Input: part model. Units: mm. Frame: model coordinates. A direction names the side the tool comes from. Round coordinates to 2 decimals unless told otherwise and drop trailing zeros. Order: outer loops, then holes, each group sorted by start corner. A loop starts at its lowest first (then second) coordinate and runs counter-clockwise, first axis right, second up.
Item 1: Reachability of faces 4 (the flat face through (0, 2.75, 3)), 5 (the flat face through (41.675, 4.435, 2.958)) from +Z, -Z, +X, -X, +Y, -Y: full face, straight path, thin tool, end or side. Return the list, or none.
Item 2: Mould query, pull axis X, two halves, no side actions, for faces 1 (the flat face through (0, -2.75, 3)), 2 (the flat face through (22, 1, 6)), 3 (the flat face through (41.438, -4.565, 2.958)). Classes: released by +X, released by -X, zero draft, split by the parting line, or undercut.
Item 3: Cut plane B-B on z = 2.8. Output: boundary loops of the cut face in (x, y), then the cut area to 3 significant figures.
Item 4: First-contact query: pin 1 (1 mm diameter, centred on x = 19, z = 4, fed in from +Y); pin 2 (3 mm diameter, centred on x = 26.5, z = 1.5, fed in from -Y); pin 3 (1.8 mm diameter, centred on x = -0.5, z = 2.5, fed in from -Y); pin 4 (1.5 mm diameter, centred on x = 5.5, y = -3.5, fed in from +Z). Flat tips, straight axial feed; report the tip coordinate or a pass-through.
Item 5: Cut plane A-A on x = 0. Output: boundary loops of the cut face in (y, z).
Item 6: Line query: L1, parallel to X at y = -2.5, z = 3.25; L2, parallel to X at y = -2.25, z = 3.8; L3, parallel to Y at x = 30, z = 1.2. Output: solid intervals per line, ascending.
Item 7: Cut plane C-C on y = -2. Output: boundary loops of the cut face in (x, z), then the cut area to 3 significant figures.
Item 8: Cut plane D-D on y = 3.5. Output: boundary loops of the cut face in (x, z), then the cut area to 3 significant figures.
Autodesk Fusion 360 part; units mm, degrees
sketch "Sketch1" plane through (0, 0, 0) normal (0, 0, 1) x (1, 0, 0)
  line L0 (38.058, -1.5) -> (4.7697, -1.5)
  line L1 (4.7697, 1.5) -> (38.0528, 1.5)
  line L2 (50, 0) -> (33.1127, 8.996)
  line L3 (33.1127, -9.004) -> (50, 0)
  line L4 (33.1127, -9.004) -> (38.058, -1.5)
  line L5 (38.0528, 1.5) -> (33.1127, 8.996)
  arc A0 (4.7697, 1.5) -> (4.7697, -1.5) centre (0, 0) ccw
  point P0 (33.1127, 8.996)
  point P1 (33.1127, -9.004)
  point P2 (39.044, -0.004)
  dimension "d1" = 10
extrude "Extrude1" add sketch "Sketch1" along normal blind 6
sketch "Sketch2" plane through (0, 0, 6) normal (0, 0, 1) x (-1, 0, 0)
  line L0 (-38.0528, -1.5) -> (-4.7697, -1.5)
  arc A0 (-4.7697, -1.5) -> (-4.7697, 1.5) centre (0, 0) ccw
  line L1 (-4.7697, 1.5) -> (-38.058, 1.5)
  line L2 (-38.058, 1.5) -> (-33.1127, 9.004)
  line L3 (-33.1127, 9.004) -> (-50, 0)
  line L4 (-50, 0) -> (-33.1127, -8.996)
  line L5 (-33.1127, -8.996) -> (-38.0528, -1.5)
  line L6 (1.75, -2.75) -> (-1.75, -2.75)
  line L7 (-1.75, -2.75) -> (-1.75, 2.75)
  line L8 (-1.75, 2.75) -> (1.75, 2.75)
  line L9 (1.75, 2.75) -> (1.75, -2.75)
  line L10 (1.75, -2.75) -> (-1.75, 2.75) construction
  line L11 (-1.75, -2.75) -> (1.75, 2.75) construction
  dimension "d9" = 3.5
  dimension "d10" = 5.5
extrude "Extrude2" cut sketch "Sketch2" against normal blind 6 contours L6 L7 L8 L9
From the geometry:
1. face 4: +Z, -Z
1. face 5: +Z, -Z, +X, +Y
2. face 1: undercut
2. face 2: zero draft
2. face 3: released by +X
3. outline: (4.77, -1.5) - (38.06, -1.5) - (33.11, -9) - (50, 0) - (33.11, 9) - (38.05, 1.5) - (4.77, 1.5) arc R5 ccw (long way) to start; hole (-1.75, -2.75) - (1.75, -2.75) - (1.75, 2.75) - (-1.75, 2.75) - close
3. area: 259 mm2
4. pin 1: stops at y = 1.5
4. pin 2: stops at y = -1.5
4. pin 3: stops at y = -5
4. pin 4: passes through
5. outline: (-5, 0) - (-2.75, 0) - (-2.75, 6) - (-5, 6) - close; (2.75, 0) - (5, 0) - (5, 6) - (2.75, 6) - close
6. L1: x = -4.33 to -1.75, 1.75 to 4.33, 37.4 to 45.31
6. L2: x = -4.47 to -1.75, 1.75 to 4.47, 37.56 to 45.78
6. L3: y = -1.5 to 1.5
7. outline: (-4.58, 0) - (-1.75, 0) - (-1.75, 6) - (-4.58, 6) - close; (1.75, 0) - (4.58, 0) - (4.58, 6) - (1.75, 6) - close; (37.73, 0) - (46.25, 0) - (46.25, 6) - (37.73, 6) - close
7. area: 85.1 mm2
8. outline: (-3.57, 0) - (3.57, 0) - (3.57, 6) - (-3.57, 6) - close; (36.73, 0) - (43.43, 0) - (43.43, 6) - (36.73, 6) - close
8. area: 83.0 mm2
